```python
from build123d import *

# Parameters (mm, degrees)
SKETCH_W            = 22.5
SKETCH_H            = 14
PAD_DEPTH           = 0.8
SKETCH001_R         = 1.1
POCKET_DEPTH        = 5
FILLET_R            = 1
SKETCH002_R         = 0.6
POCKET001_DEPTH     = 5
LINEARPATTERN_COUNT = 4
LINEARPATTERN_PITCH = 3.666667


with BuildPart() as part:
    # Sketch → Pad (new body)
    with BuildSketch(Plane.XZ):
        with Locations((11.25, 7)):
            Rectangle(SKETCH_W, SKETCH_H)
    extrude(amount=PAD_DEPTH)

    # Sketch001 (on Face6 of Pad) → Pocket (cut)
    with BuildSketch(Plane.XZ.offset(0.8)):
        with Locations((3, 11)):
            Circle(SKETCH001_R)
        with Locations((3, 3)):
            Circle(SKETCH001_R)
    extrude(amount=-POCKET_DEPTH, mode=Mode.SUBTRACT)

    # Fillet
    fillet_edges = [part.edges().sort_by_distance(p)[0] for p in [
        (0, -0.4, 14),
        (22.5, -0.4, 14),
        (22.5, -0.4, 0),
        (0, -0.4, 0),
    ]]
    fillet(fillet_edges, radius=FILLET_R)

    # Sketch002 (on Face5 of Fillet) → Pocket001 (cut)
    with BuildSketch(Plane.XZ.offset(0.8)):
        with Locations((7.5, 11)):
            Circle(SKETCH002_R)
        with Locations((7.5, 3)):
            Circle(SKETCH002_R)
    pocket001 = extrude(amount=-POCKET001_DEPTH, mode=Mode.SUBTRACT)

    # LinearPattern: Pocket001 ×4
    with Locations(*[(i * LINEARPATTERN_PITCH, 0, 0) for i in range(1, LINEARPATTERN_COUNT)]):
        add(pocket001, mode=Mode.SUBTRACT)


solid = part.part
```
CAD build for the part. Positions are in the model's coordinates, mm. Coordinates: 2 decimals unless noted, no trailing zeros. Write each loop counter-clockwise with the first axis right and the second up, starting at its lowest first coordinate (ties: lowest second). Pieces come first, ordered by that corner, then holes. Notation, with made-up numbers: (-9, 70) -> (15, 70) arc R17 ccw to (15, 97) -> close; hole circle Ø7 at (60, 4). An arc over 180 degrees is marked (long way). Use CSV: the item, a comma, the result in double quotes. Start each with the question number.
Item 1: Two-plate mould, pull along Z, no slides. Class faces 1 (the cylindrical face through (0.285, -0.406, 0.301)), 2 (the cylindrical face through (0.285, -0.406, 13.699)), 3 (the cylindrical face through (7.78, -0.41, 10.47)): +Z half, -Z half, draft (parallel to the pull), parting line (faces both ways), or undercut.
Item 2: Band-saw the part on B-B, the plane z = 3. Write the cut outline in (x, y).
Item 3: Drop flat-ended pins along their axis: P1, Ø1.9, axis at x = 7.5, z = 3, coming from the +Y side; P2, Ø0.7, axis at x = 14.83, z = 3, coming from the +Y side. Give the stop position or say it passes through.
Item 4: Wall check: probe 1 along Z at (x, y) = (3, -0.5); probe 2 along Z at (x, y) = (18.5, -0.6); probe 3 along X at (y, z) = (-0.25, 10.75). Give the ranges that are in metal, low to high.
Item 5: Band-saw the part on C-C, the plane y = -0.35. Give the number of separate pieces and of enclosed holes in the cut face, plus the area to 3 significant figures.
Item 6: Band-saw the part on A-A, the plane x = 7.5. Write the cut outline in (y, z), plus the area to 3 significant figures.
Response values:
1,face 1,"-Z half"
1,face 2,"+Z half"
1,face 3,"undercut"
2,outline,"(0, -0.8) -> (1.9, -0.8) -> (1.9, 0) -> (0, 0) -> close; (4.1, -0.8) -> (6.9, -0.8) -> (6.9, 0) -> (4.1, 0) -> close; (8.1, -0.8) -> (10.57, -0.8) -> (10.57, 0) -> (8.1, 0) -> close; (11.77, -0.8) -> (14.23, -0.8) -> (14.23, 0) -> (11.77, 0) -> close; (15.43, -0.8) -> (17.9, -0.8) -> (17.9, 0) -> (15.43, 0) -> close; (19.1, -0.8) -> (22.5, -0.8) -> (22.5, 0) -> (19.1, 0) -> close"
3,P1,"stops at y = 0"
3,P2,"passes through"
4,probe 1,"z = 0 to 1.9, 4.1 to 9.9, 12.1 to 14"
4,probe 2,"z = 0 to 2.4, 3.6 to 10.4, 11.6 to 14"
4,probe 3,"x = 0 to 1.93, 4.07 to 6.95, 8.05 to 10.62, 11.71 to 14.29, 15.38 to 17.95, 19.05 to 22.5"
5,separate pieces,"1"
5,enclosed holes,"10"
5,area,"297 mm2"
6,outline,"(-0.8, 0) -> (0, 0) -> (0, 2.4) -> (-0.8, 2.4) -> close; (-0.8, 3.6) -> (0, 3.6) -> (0, 10.4) -> (-0.8, 10.4) -> close; (-0.8, 11.6) -> (0, 11.6) -> (0, 14) -> (-0.8, 14) -> close"
6,area,"9.28 mm2"
